Here's how the part is built. I have some questions about the finished solid (model axes, mm). A direction names the side the tool comes from. Round coordinates to 2 decimals unless told otherwise and drop trailing zeros. Order: outer loops, then holes, each group sorted by start corner. A loop starts at its lowest first (then second) coordinate and runs counter-clockwise, first axis right, second up. Notation, with made-up numbers: M -12.5,-12.75 L 28.5,-12.75 A25 cw 28.5,6.25 Z; hole C -5.75,65 d5. An arc over 180 degrees is marked long. Write item = value, one per line. Start each with the question number.
Item 1: I'm going to push a flat-ended pin straight in: P1, Ø1.5, axis at x = -11, y = -11, coming from the -Z side. Where does the tip first touch, or does it pass through?
Item 2: Please list where these lines run through material, in increasing order: L1, parallel to Y at x = -11, z = 2.6; L2, parallel to X at y = -6.5, z = 1.95; L3, parallel to Y at x = 11, z = 2.5.
Item 3: I want a section at C-C, the plane z = 2.45. List the corners of the cut face in (x, y) for me, plus the area to 3 significant figures.
Item 4: I want a section at D-D, the plane y = 13. List the corners of the cut face in (x, z) for me.
Item 5: I want a section at A-A, the plane y = 1. List the corners of the cut face in (x, z) for me.
Item 6: We'd pull the mould along X, two halves only. Please class faces 4 (the face through (-11.921, -11.845, 2.493)), 5 (the face through (-20, -0.2, 2.5)), 6 (the face through (-0.21, 19.4, 0.57)): pulls with the +X half, pulls with the -X half, needs draft (parallel to the pull), parting line crosses it, or undercut.
Item 7: I want a section at B-B, the plane x = -13. List the corners of the cut face in (y, z) for me.
Item 8: For faces 1 (the face through (-18.57, 18.5, 2.51)), 2 (the face through (-14, 0, 2)), 3 (the face through (-3.5, 0.1, 0.5)), which set-ups out of +Z, -Z, +X, -X, +Y, -Y let a thin tool reach every point of the face, with its end or its side?
```python
from build123d import *

# Parameters (mm, degrees)
SKETCH_W        = 40
SKETCH_H        = 40
PAD_DEPTH       = 3
SKETCH001_R     = 2.5
POCKET_DEPTH    = 2
SKETCH002_R     = 1.25
POCKET001_DEPTH = 1
FILLET_R        = 5
SKETCH003_W     = 10
SKETCH003_H     = 14
POCKET002_DEPTH = 3
CHAMFER_SIZE    = 1
FILLET002_R     = 2


with BuildPart() as part:
    # Sketch → Pad (new body)
    with BuildSketch(Plane.XY):
        Rectangle(SKETCH_W, SKETCH_H)
    extrude(amount=PAD_DEPTH)

    # Sketch001 (on Face5 of Pad) → Pocket (cut)
    with BuildSketch(Plane(origin=(0, 0, 0), x_dir=(1, 0, 0), z_dir=(0, 0, -1))):
        with Locations((-11, 11)):
            Circle(SKETCH001_R)
        with Locations((11, -11)):
            Circle(SKETCH001_R)
    extrude(amount=-POCKET_DEPTH, mode=Mode.SUBTRACT)

    # Sketch002 (on Face9 of Pocket) → Pocket001 (cut)
    with BuildSketch(Plane(origin=(0, 0, 2), x_dir=(1, 0, 0), z_dir=(0, 0, -1))):
        with Locations((-11, 11)):
            Circle(SKETCH002_R)
        with Locations((11, -11)):
            Circle(SKETCH002_R)
    extrude(amount=-POCKET001_DEPTH, mode=Mode.SUBTRACT)

    # Fillet
    fillet_edges = [part.edges().sort_by_distance(p)[0] for p in [
        (-20, -20, 1.5),
        (-20, 20, 1.5),
        (20, 20, 1.5),
        (20, -20, 1.5),
    ]]
    fillet(fillet_edges, radius=FILLET_R)

    # Sketch003 (on Face2 of Fillet) → Pocket002 (cut)
    with BuildSketch(Plane(origin=(0, 0, 0), x_dir=(1, 0, 0), z_dir=(0, 0, -1))):
        with Locations((-9, 0)):
            Rectangle(SKETCH003_W, SKETCH003_H)
    extrude(amount=-POCKET002_DEPTH, mode=Mode.SUBTRACT)

    # Chamfer
    chamfer_edges = [part.edges().sort_by_distance(p)[0] for p in [
        (-9, -7, 0),
        (-14, 0, 0),
        (-9, 7, 0),
        (-4, 0, 0),
    ]]
    chamfer(chamfer_edges, length=CHAMFER_SIZE)

    # Fillet002
    fillet002_edges = [part.edges().sort_by_distance(p)[0] for p in [
        (-18.535534, -18.535534, 0),
        (-20, 0, 0),
        (0, -20, 0),
        (18.535534, -18.535534, 0),
        (20, 0, 0),
        (18.535534, 18.535534, 0),
        (0, 20, 0),
        (-18.535534, 18.535534, 0),
    ]]
    fillet(fillet002_edges, radius=FILLET002_R)


solid = part.part
```
Filled in:
q1.P1 = through
q2.L1 = -20 to -12.25, -9.75 to -7, 7 to 20
q2.L2 = -20 to -14, -4 to 20
q2.L3 = -20 to 9.75, 12.25 to 20
q3.outline = M -20,-15 A5 ccw -15,-20 L 15,-20 A5 ccw 20,-15 L 20,15 A5 ccw 15,20 L -15,20 A5 ccw -20,15 Z; hole M -14,-7 L -4,-7 L -4,7 L -14,7 Z; hole C -11,-11 d2.5; hole C 11,11 d2.5
q3.area = 1,430 mm^2
q4.outline = M -20,2 A2 ccw -18,0 L 9.5,0 L 9.5,2 L 12.5,2 L 12.5,0 L 18,0 A2 ccw 20,2 L 20,3 L -20,3 Z
q5.outline = M -20,2 A2 ccw -18,0 L -15,0 L -14,1 L -14,3 L -20,3 Z; M -4,1 L -3,0 L 18,0 A2 ccw 20,2 L 20,3 L -4,3 Z
q6.face_4 = undercut
q6.face_5 = pulls with the -X half
q6.face_6 = needs draft
q7.outline = M -20,2 A2 ccw -18,0 L -12.5,0 L -12.5,2 L -9.5,2 L -9.5,0 L -8,0 L -7,1 L -7,3 L -20,3 Z; M 7,1 L 8,0 L 18,0 A2 ccw 20,2 L 20,3 L 7,3 Z
q8.face_1 = +Z, -Z, -X, +Y
q8.face_2 = +Z, -Z
q8.face_3 = -Z
